from build123d import *

# Parameters (mm, degrees)
SKETCH1_W                                       = 30
SKETCH1_H                                       = 180
BOSS_EXTRUDE1_DEPTH                             = 8
CHAMFER1_SIZE                                   = 3
CBORE_FOR_M5_SOCKET_HEAD_CAP_SCREW1_D           = 5.5
CBORE_FOR_M5_SOCKET_HEAD_CAP_SCREW1_CBORE_D     = 10
CBORE_FOR_M5_SOCKET_HEAD_CAP_SCREW1_CBORE_DEPTH = 5
CBORE_FOR_M5_SOCKET_HEAD_CAP_SCREW2_D           = 5.5
CBORE_FOR_M5_SOCKET_HEAD_CAP_SCREW2_CBORE_D     = 10
CBORE_FOR_M5_SOCKET_HEAD_CAP_SCREW2_CBORE_DEPTH = 5


with BuildPart() as part:
    # Sketch1 → Boss-Extrude1 (new body)
    with BuildSketch(Plane(origin=(0, 0, 0), x_dir=(1, 0, 0), z_dir=(0, 1, 0))):
        with Locations((15, 0)):
            Rectangle(SKETCH1_W, SKETCH1_H)
    extrude(amount=BOSS_EXTRUDE1_DEPTH)

    # Chamfer1
    chamfer1_edges = [part.edges().sort_by_distance(p)[0] for p in [
        (30, 4, 90),
        (0, 4, 90),
        (0, 4, -90),
        (30, 4, -90),
    ]]
    chamfer(chamfer1_edges, length=CHAMFER1_SIZE)

    # CBORE for M5 Socket Head Cap Screw1 (through all)
    with Locations(Plane(origin=(0, 8, 0), x_dir=(-1, 0, 0), z_dir=(0, 1, 0))):
        with Locations((-6, -80), (-6, 80), (-24, 80), (-24, -80)):
            CounterBoreHole(CBORE_FOR_M5_SOCKET_HEAD_CAP_SCREW1_D / 2, CBORE_FOR_M5_SOCKET_HEAD_CAP_SCREW1_CBORE_D / 2, CBORE_FOR_M5_SOCKET_HEAD_CAP_SCREW1_CBORE_DEPTH)

    # CBORE for M5 Socket Head Cap Screw2 (through all)
    with Locations(Plane.XZ):
        with Locations((6, 30), (6, -30), (24, -30), (24, 30)):
            CounterBoreHole(CBORE_FOR_M5_SOCKET_HEAD_CAP_SCREW2_D / 2, CBORE_FOR_M5_SOCKET_HEAD_CAP_SCREW2_CBORE_D / 2, CBORE_FOR_M5_SOCKET_HEAD_CAP_SCREW2_CBORE_DEPTH)


solid = part.part
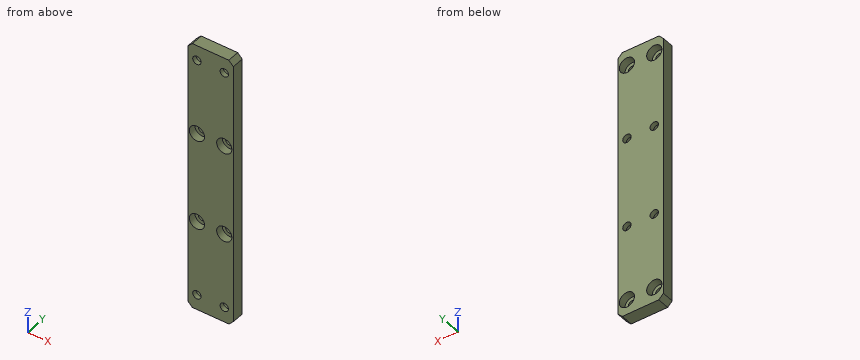
Could you check a few things on this model? Use its own coordinates, in mm. Round coordinates to 2 decimals unless told otherwise and drop trailing zeros. Write each loop counter-clockwise with the first axis right and the second up, starting at its lowest first coordinate (ties: lowest second). Pieces come first, ordered by that corner, then holes. Notation, with made-up numbers: (52, 45.25) - (83, 45.25) arc R24 cw to (83, 71.25) - close; hole circle Ø2 at (66, 30). An arc over 180 degrees is marked (long way). Use a Markdown table: item, result.
Q1. I want a section at B-B (x = 24). Count the separate pieces of the cut face and the enclosed holes in it, plus the area to 3 significant figures.
Output values:
| item | result |
|---|---|
| separate pieces | 5 |
| enclosed holes | 0 |
| area | 1,170 mm2 |
Q2. I want a section at A-A (z = -30). List the corners of the cut face in (x, y) for me.
Output values:
| item | result |
|---|---|
| outline | (0, 0) - (1, 0) - (1, 5) - (3.25, 5) - (3.25, 8) - (0, 8) - close; (8.75, 5) - (11, 5) - (11, 0) - (19, 0) - (19, 5) - (21.25, 5) - (21.25, 8) - (8.75, 8) - close; (26.75, 5) - (29, 5) - (29, 0) - (30, 0) - (30, 8) - (26.75, 8) - close |
Q3. Please list where these lines run through material, in increasing order: L1, parallel to X at y = 2.25, z = -30.5; L2, parallel to Z at x = 6, y = 1.7; L3, parallel to Z at x = 6, y = 6.75.
Output values:
| item | result |
|---|---|
| L1 | 0 to 1.03, 10.97 to 19.03, 28.97 to 30 |
| L2 | -90 to -82.75, -77.25 to -35, -25 to 25, 35 to 77.25, 82.75 to 90 |
| L3 | -90 to -85, -75 to -32.75, -27.25 to 27.25, 32.75 to 75, 85 to 90 |
Q4. For pin 1 (6.5 mm diameter, centred on x = 6, z = -30, fed in from -Y); pin 2 (3 mm diameter, centred on x = 25, z = -78.5, fed in from +Y), each with a flat end and sliding along its axis, tell me the tip position at first contact or that it passes through.
Output values:
| item | result |
|---|---|
| pin 1 | y = 5 |
| pin 2 | y = 3 |
